For this review, take the finished solid that the model builds, in its own axes (mm). Give positions to 0.01 mm unless a question says otherwise; leave off trailing zeros. Loops run counter-clockwise (first coordinate to the right, second up) from the corner with the lowest first, then second, coordinate; pieces in that order, holes last.
Autodesk Inventor part; units mm, degrees
ref_plane "YZ Plane" through (0, 0, 0) normal (1, 0, 0) x (0, 1, 0)
ref_plane "XZ Plane" through (0, 0, 0) normal (0, 1, 0) x (-1, 0, 0)
ref_plane "XY Plane" through (0, 0, 0) normal (0, 0, 1) x (1, 0, 0)
sketch "Sketch1" plane through (0, 0, 0) normal (0, 0, 1) x (1, 0, 0)
  line L0 (-75, 33) -> (75, 33)
  line L1 (75, 33) -> (75, -33)
  line L2 (75, -33) -> (-75, -33)
  line L3 (-75, -33) -> (-75, 33)
  point P0 (0, 0)
  point P1 (0, 33)
  point P2 (-75, 0)
  dimension "d0" = 150
  dimension "d1" = 66
extrude "Extrusion1" add sketch "Sketch1" along normal blind 8
sketch "Sketch4" plane through (0, 0, 8) normal (0, 0, 1) x (1, 0, 0)
  circle A0 centre (-60, -25) radius 2.25
  circle A1 centre (-60, 25) radius 2.25
  line L0 (-75, 33) -> (-75, -33)
  line L1 (-75, -33) -> (75, -33)
  line L2 (75, 33) -> (-75, 33)
  circle A2 centre (-60, 0) radius 2.25
  circle A3 centre (-28, -25) radius 2.25
  circle A4 centre (-28, 0) radius 2.25
  circle A5 centre (-28, 25) radius 2.25
  circle A6 centre (60, -25) radius 2.25
  line L3 (75, -33) -> (75, 33)
  circle A7 centre (60, 0) radius 2.25
  circle A8 centre (60, 25) radius 2.25
  circle A9 centre (28, -25) radius 2.25
  circle A10 centre (28, 0) radius 2.25
  circle A11 centre (28, 25) radius 2.25
  circle A12 centre (0, -25) radius 2.25
  circle A13 centre (0, 25) radius 2.25
  point P0 (0, 0)
  point P1 (-75, 0)
  point P2 (-75, 0)
  dimension "d19" = 4.5
  dimension "d20" = 15
  dimension "d21" = 8
  dimension "d22" = 8
  dimension "d23" = 32
  dimension "d24" = 15
  dimension "d26" = 32
extrude "Extrusion4" cut sketch "Sketch4" against normal through all contours A0 | A1 | A2 | A3 | A4 | A5 | A6 | A7 | A8 | A9 | A10 | A11 | A12 | A13
equation "\"d22\" = d21"
equation "\"d24\" = d20"
equation "\"d26\" = d23"
properties part number "0005-10-022 fixare rulmenti"
Q1. Consider section C-C on x = 0. Give the boundary of the cut face in (y, z).
Answers:
outline: (-33, 0) - (-27.25, 0) - (-27.25, 8) - (-33, 8) - close; (-22.75, 0) - (22.75, 0) - (22.75, 8) - (-22.75, 8) - close; (27.25, 0) - (33, 0) - (33, 8) - (27.25, 8) - close
Q2. For probe 1 along Y at (x, z) = (-60, 5.5); probe 2 along Y at (x, z) = (-30, 1); probe 3 along X at (y, z) = (-26.5, 4.5), list the stretches that pass through material, from the lowest coordinate up.
Answers:
probe 1: y = -33 to -27.25, -22.75 to -2.25, 2.25 to 22.75, 27.25 to 33
probe 2: y = -33 to -26.03, -23.97 to -1.03, 1.03 to 23.97, 26.03 to 33
probe 3: x = -75 to -61.68, -58.32 to -29.68, -26.32 to -1.68, 1.68 to 26.32, 29.68 to 58.32, 61.68 to 75
Q3. For pin 1 Ø2.5 at (x, y) = (28, 0) entering from -Z; pin 2 Ø6 at (x, y) = (0, -25) entering from -Z, all flat-tipped, find the tip position at first contact; note any pin that passes through.
Answers:
pin 1: passes through
pin 2: stops at z = 0
Q4. Mouldability with a two-part tool opening along Y and no side actions: class faces 1 (the cylindrical face through (29.038, 23.004, 4.056)), 2 (the flat face through (75, 0, 4)), 3 (the flat face through (-1, 33, 4)), 4 (the cylindrical face through (29.038, -26.996, 4.056)) as +Y half, -Y half, draft (parallel to the pull), parting line (faces both ways), or undercut.
Answers:
face 1: undercut
face 2: draft
face 3: +Y half
face 4: undercut
Q5. Consider section B-B on y = 25. Give the boundary of the cut face in (x, z), plus the area to 3 significant figures.
Answers:
outline: (-75, 0) - (-62.25, 0) - (-62.25, 8) - (-75, 8) - close; (-57.75, 0) - (-30.25, 0) - (-30.25, 8) - (-57.75, 8) - close; (-25.75, 0) - (-2.25, 0) - (-2.25, 8) - (-25.75, 8) - close; (2.25, 0) - (25.75, 0) - (25.75, 8) - (2.25, 8) - close; (30.25, 0) - (57.75, 0) - (57.75, 8) - (30.25, 8) - close; (62.25, 0) - (75, 0) - (75, 8) - (62.25, 8) - close
area: 1,020 mm2
Q6. Consider section A-A on x = 28. Give the boundary of the cut face in (y, z), plus the area to 3 significant figures.
Answers:
outline: (-33, 0) - (-27.25, 0) - (-27.25, 8) - (-33, 8) - close; (-22.75, 0) - (-2.25, 0) - (-2.25, 8) - (-22.75, 8) - close; (2.25, 0) - (22.75, 0) - (22.75, 8) - (2.25, 8) - close; (27.25, 0) - (33, 0) - (33, 8) - (27.25, 8) - close
area: 420 mm2
Q7. Consider section D-D on z = 4.75. Count the separate pieces of the cut face and the enclosed holes in it, plus the area to 3 significant figures.
Answers:
separate pieces: 1
enclosed holes: 14
area: 9,680 mm2
